The model under review builds one solid part; all positions refer to its coordinate system, in mm. Face numbers are marked on the shaded views. A direction names the side the tool comes from. Coordinates: 2 decimals unless noted, no trailing zeros. Write each loop counter-clockwise with the first axis right and the second up, starting at its lowest first coordinate (ties: lowest second). Pieces come first, ordered by that corner, then holes. Notation, with made-up numbers: (1.5, 0.5) - (47.5, 0.5) arc R25 cw to (47.5, 21.5) - close; hole circle Ø3 at (23, 2). An arc over 180 degrees is marked (long way). Put each result on its own line as item: value. Start each with the question number.
Item 1: Consider section B-B on z = 0. Give the boundary of the cut face in (x, y) (3 decimals), then the cut area to 3 significant figures.
Item 2: Consider section A-A on y = 0. State how many separate pieces and enclosed holes the cut face has, then the cut area to 3 significant figures.
Item 3: Consider section C-C on x = -4. Give the boundary of the cut face in (y, z), then the cut area to 3 significant figures.
Item 4: Machinability: for the marked faces 1, 2 and 3, which of the approach directions +Z, -Z, +X, -X, +Y, -Y give a long, thin tool a straight path to every point of the face, cutting with its end or side? Answer none if there is none.
Item 5: To check wall thickness, follow L1, parallel to Z at x = -6, y = 0; L2, parallel to Z at x = -15, y = 0 (3 decimals); L3, parallel to Z at x = -6.5, y = -1. State the ranges of each line that lie inside material, in increasing order. Write a range as [from, to].
Item 6: For pin 1 (5 mm diameter, centred on y = 29.5, z = -12.5, fed in from -X); pin 2 (5 mm diameter, centred on x = -5.5, z = 28.5, fed in from +Y); pin 3 (6 mm diameter, centred on x = -8.5, y = 9.5, fed in from -Z), all flat-tipped, find the tip position at first contact; note any pin that passes through.
Item 7: Mouldability with a two-part tool opening along Z and no side actions: class the marked faces 4, 5 and 6 as pulls with the +Z half, pulls with the -Z half, needs draft (parallel to the pull), parting line crosses it, or undercut.
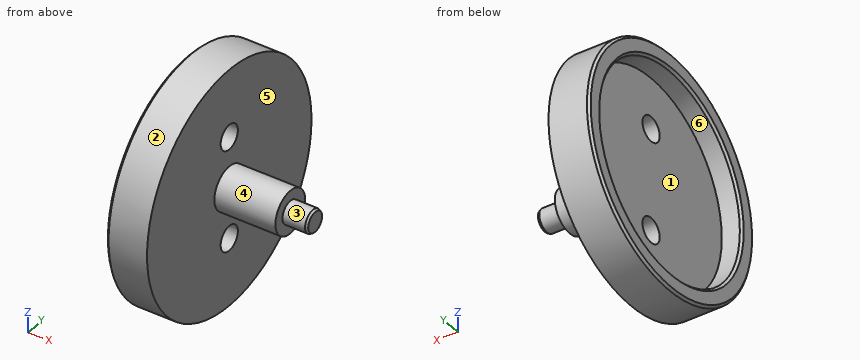
```python
from build123d import *

# Parameters (mm, degrees)
F0_R     = 52.5
F1_DEPTH = 18
F2_R     = 45.125
F3_DEPTH = 9
F4_SIZE  = 1
F5_R     = 9.5
F6_DEPTH = 27
F7_R     = 5
F8_DEPTH = 11
F9_SIZE2 = 0.5773502692
F9_SIZE  = 1
F11_D    = 11


with BuildPart() as f1:
    # F0 (on Right) → F1 (new body)
    with BuildSketch(Plane.YZ):
        Circle(F0_R)
    extrude(amount=-F1_DEPTH)

    # F2 (on face) → F3 (cut)
    with BuildSketch(Plane(origin=(-18, 0, 0), x_dir=(0, -1, 0), z_dir=(-1, 0, 0))):
        Circle(F2_R)
    extrude(amount=-F3_DEPTH, mode=Mode.SUBTRACT)

    # F4
    f4_edges = [f1.edges().sort_by_distance(p)[0] for p in [
        (-18, -52.5, 0),
        (-18, 45.125, 0),
    ]]
    chamfer(f4_edges, length=F4_SIZE)

    # F5 (on face) → F6 (join)
    with BuildSketch(Plane.YZ):
        Circle(F5_R)
    extrude(amount=F6_DEPTH)

    # F7 (on face) → F8 (join)
    with BuildSketch(Plane.YZ.offset(27)):
        Circle(F7_R)
    extrude(amount=F8_DEPTH)

    # F9
    f9_edges = [f1.edges().sort_by_distance(p)[0] for p in [
        (38, -5, 0),
    ]]
    f9_side = f1.faces().sort_by_distance((32.5, -5, 0))[0]
    chamfer(f9_edges, length=F9_SIZE, length2=F9_SIZE2, reference=f9_side)

    # F11 (through all)
    with Locations(Plane.YZ):
        with Locations((0, -22.5), (0, 22.5)):
            Hole(F11_D / 2)


solid = f1.part
```
Report:
1. outline: (-18, -51.5) - (-17, -52.5) - (0, -52.5) - (0, -9.5) - (27, -9.5) - (27, -5) - (37, -5) - (38, -4.423) - (38, 4.423) - (37, 5) - (27, 5) - (27, 9.5) - (0, 9.5) - (0, 52.5) - (-17, 52.5) - (-18, 51.5) - (-18, 46.125) - (-17, 45.125) - (-9, 45.125) - (-9, -45.125) - (-17, -45.125) - (-18, -46.125) - close
1. area: 1,700 mm²
2. separate pieces: 3
2. enclosed holes: 0
2. area: 1,500 mm²
3. outline: circle Ø105 at (0, 0); hole circle Ø11 at (0, -22.5); hole circle Ø11 at (0, 22.5)
3. area: 8,470 mm²
4. face 1: -X
4. face 2: +X, -X
4. face 3: +X
5. L1: [-52.5, -28], [-17, 17], [28, 52.5]
5. L2: [-52.5, -45.125], [45.125, 52.5]
5. L3: [-52.49, -27.91], [-17.09, 17.09], [27.91, 52.49]
6. pin 1: x = -9
6. pin 2: y = 45.61
6. pin 3: z = -52.1
7. face 4: parting line crosses it
7. face 5: needs draft
7. face 6: undercut
